from build123d import *

# Parameters (mm, degrees)
F0_W         = 70.9387809038
F0_H         = 53.9411939681
F1_DEPTH     = 38.1
F2_T         = -2.54
F3_R         = 5.08
F4_T1_DEPTH  = 43.7811939681
F4_T3_DEPTH  = 45.72
F4_S7_W      = 5.08
F4_S7_H      = 5.08
F4_T8_DEPTH  = 5.08
F4_S13_W     = 5.08
F4_S13_H     = 5.08
F4_T14_DEPTH = 5.08
F4_T18_ANGLE = 90
F4_T20_ANGLE = 90


# Not quite as in the source:
# - a fillet or chamfer that OpenCascade refuses, or shapes differently, is made with other operations: its cross-section is extruded or revolved along the edge and cut away or added


with BuildPart() as f1:
    # F0 (on Top) → F1 (new body)
    with BuildSketch(Plane.XY):
        Rectangle(F0_W, F0_H)
    extrude(amount=F1_DEPTH)

    # F2
    f2_openings = [f1.faces().sort_by_distance(p)[0] for p in [
        (0, 0, 38.1),
    ]]
    offset(amount=F2_T, openings=f2_openings)

    # F3
    f3_edges = [f1.edges().sort_by_distance(p)[0] for p in [
        (0, 26.970597, 0),
        (0, -26.970597, 0),
        (-35.46939, 26.970597, 19.05),
        (35.46939, -26.970597, 19.05),
    ]]
    fillet(f3_edges, radius=F3_R)

    # F4: fillet of radius 5.08 on 3 edges, made by hand

    # F4_s2 → F4_t1 (cut)
    with BuildSketch(Plane.XZ.offset(-21.890596984)):
        with BuildLine():
            ThreePointArc((30.3893904519, 0), (33.9814929003, 1.4878975516), (35.4693904519, 5.08))
            Line((35.4693904519, 5.08), (35.4693904519, 0))
            Line((35.4693904519, 0), (30.3893904519, 0))
        make_face()
        with BuildLine():
            ThreePointArc((-35.4693904519, 5.08), (-33.9814929003, 1.4878975516), (-30.3893904519, 0))
            Line((-30.3893904519, 0), (-35.4693904519, 0))
            Line((-35.4693904519, 0), (-35.4693904519, 5.08))
        make_face()
    extrude(amount=F4_T1_DEPTH, mode=Mode.SUBTRACT)

    # F4_s4 → F4_t3 (cut)
    with BuildSketch(Plane.XY.offset(5.08)):
        with BuildLine():
            ThreePointArc((-30.3893904519, -26.970596984), (-33.9814929003, -25.4826994325), (-35.4693904519, -21.890596984))
            Line((-35.4693904519, -21.890596984), (-35.4693904519, -26.970596984))
            Line((-35.4693904519, -26.970596984), (-30.3893904519, -26.970596984))
        make_face()
        with BuildLine():
            ThreePointArc((35.4693904519, 21.890596984), (33.9814929003, 25.4826994325), (30.3893904519, 26.970596984))
            Line((30.3893904519, 26.970596984), (35.4693904519, 26.970596984))
            Line((35.4693904519, 26.970596984), (35.4693904519, 21.890596984))
        make_face()
    extrude(amount=F4_T3_DEPTH, mode=Mode.SUBTRACT)


with BuildPart() as f4_tool6:
    # F4_s7 → F4_t8 (new body)
    with BuildSketch(Plane.YZ.offset(-30.3893904519)):
        with Locations((24.430596984, 2.54)):
            Rectangle(F4_S7_W, F4_S7_H)
    extrude(amount=-F4_T8_DEPTH)

    # F4_s9 → F4_t10 (revolve, cut)
    with BuildSketch(Plane(origin=(-30.3893904519, 21.890596984, 5.08), x_dir=(0, -0.7071067812, 0.7071067812), z_dir=(0, -0.7071067812, -0.7071067812))):
        with BuildLine():
            ThreePointArc((0, -5.08), (5.08, 0), (0, 5.08))
            Line((0, 5.08), (0, -5.08))
        make_face()
    revolve(axis=Axis((-30.3893904519, 21.890596984, 5.08), (-1, 0, 0)), mode=Mode.SUBTRACT)


with BuildPart() as f1_1:
    add(f1.part)

    # F4_t5: cut F4_tool6
    add(f4_tool6.part, mode=Mode.SUBTRACT)


with BuildPart() as f4_tool12:
    # F4_s13 → F4_t14 (new body)
    with BuildSketch(Plane.XY.offset(5.08)):
        with Locations((32.9293904519, -24.430596984)):
            Rectangle(F4_S13_W, F4_S13_H)
    extrude(amount=-F4_T14_DEPTH)

    # F4_s15 → F4_t16 (revolve, cut)
    with BuildSketch(Plane(origin=(30.3893904519, -21.890596984, 5.08), x_dir=(-0.7071067812, 0.7071067812, 0), z_dir=(-0.7071067812, -0.7071067812, 0))):
        with BuildLine():
            ThreePointArc((0, -5.08), (5.08, 0), (0, 5.08))
            Line((0, 5.08), (0, -5.08))
        make_face()
    revolve(axis=Axis((30.3893904519, -21.890596984, 5.08), (0, 0, -1)), mode=Mode.SUBTRACT)


with BuildPart() as f1_2:
    add(f1_1.part)

    # F4_t11: cut F4_tool12
    add(f4_tool12.part, mode=Mode.SUBTRACT)

    # F4_s17 → F4_t18 (revolve, cut)
    with BuildSketch(Plane.XY.offset(5.08)):
        with BuildLine():
            ThreePointArc((-35.4693904519, -21.890596984), (-33.9814929003, -25.4826994325), (-30.3893904519, -26.970596984))
            Line((-30.3893904519, -26.970596984), (-35.4693904519, -26.970596984))
            Line((-35.4693904519, -26.970596984), (-35.4693904519, -21.890596984))
        make_face()
    revolve(axis=Axis((-35.4693904519, -21.890596984, 5.08), (1, 0, 0)), revolution_arc=F4_T18_ANGLE, mode=Mode.SUBTRACT)

    # F4_s19 → F4_t20 (revolve, cut)
    with BuildSketch(Plane.XY.offset(5.08)):
        with BuildLine():
            ThreePointArc((35.4693904519, 21.890596984), (33.9814929003, 25.4826994325), (30.3893904519, 26.970596984))
            Line((30.3893904519, 26.970596984), (35.4693904519, 26.970596984))
            Line((35.4693904519, 26.970596984), (35.4693904519, 21.890596984))
        make_face()
    revolve(axis=Axis((35.4693904519, 21.890596984, 5.08), (-1, 0, 0)), revolution_arc=F4_T20_ANGLE, mode=Mode.SUBTRACT)


solid = f1_2.part
Geometry check sheet. Reference: the model listing, model coordinates, mm. A direction names the side the tool comes from. Coordinates: 2 decimals unless noted, no trailing zeros. Order: outer loops, then holes, each group sorted by start corner. A loop starts at its lowest first (then second) coordinate and runs counter-clockwise, first axis right, second up. Notation, with made-up numbers: (-33, 73) -> (15, 73) arc R20 ccw to (15, 110) -> close; hole circle Ø9 at (68.5, 15). An arc over 180 degrees is marked (long way). Use a Markdown table: item, result. Add a question column.
1. Mould release check, pull along X, two halves, no side actions. Record for faces 3 (the face through (-34.021, 0.306, 1.528)), 4 (the face through (34.021, 25.443, 21.359)), 5 (the face through (32.929, 0, 20)): pulls with the +X half, pulls with the -X half, needs draft (parallel to the pull), parting line crosses it, or undercut.
2. Set-up check for faces 1 (the face through (-34.021, 25.443, 21.821)), 2 (the face through (0, 0, 2.54)): record each of +Z, -Z, +X, -X, +Y, -Y from which the full face is reachable in a straight line by a thin tool's end or side.
3. Go/stop test with a flat-tipped pin: pin 1 Ø1.5 at (x, y) = (-3.5, -6) entering from +Z. Record where the tip stops, or that it passes through.
4. Cross-section at C-C (y = -11.5). Enter the section's corners in (x, z), and give its area (3 significant figures).
5. Cross-section at B-B (x = -23). Enter the section's corners in (y, z).
6. Cross-section at A-A (z = 25.5). Enter the section's corners in (x, y), and give its area (3 significant figures).
7. Material ranges on L1, parallel to Y at x = 1, z = 16; L2, parallel to X at y = -15.5, z = 35; L3, parallel to Z at x = -29, y = 9, recorded low to high.
Filled sheet:
| question | item | result |
|---|---|---|
| 1 | face 3 | pulls with the -X half |
| 1 | face 4 | pulls with the +X half |
| 1 | face 5 | undercut |
| 2 | face 1 | +Z, -Z, -X, +Y |
| 2 | face 2 | +Z |
| 3 | pin 1 | z = 2.54 |
| 4 | outline | (-35.47, 5.08) arc R5.08 ccw to (-30.39, 0) -> (30.39, 0) arc R5.08 ccw to (35.47, 5.08) -> (35.47, 38.1) -> (32.93, 38.1) -> (32.93, 2.54) -> (-32.93, 2.54) -> (-32.93, 38.1) -> (-35.47, 38.1) -> close |
| 4 | area | 350 mm2 |
| 5 | outline | (-26.97, 5.08) arc R5.08 ccw to (-21.89, 0) -> (21.89, 0) arc R5.08 ccw to (26.97, 5.08) -> (26.97, 38.1) -> (24.43, 38.1) -> (24.43, 2.54) -> (-24.43, 2.54) -> (-24.43, 38.1) -> (-26.97, 38.1) -> close |
| 6 | outline | (-35.47, -21.89) arc R5.08 ccw to (-30.39, -26.97) -> (30.39, -26.97) arc R5.08 ccw to (35.47, -21.89) -> (35.47, 21.89) arc R5.08 ccw to (30.39, 26.97) -> (-30.39, 26.97) arc R5.08 ccw to (-35.47, 21.89) -> close; hole (-32.93, -24.43) -> (32.93, -24.43) -> (32.93, 24.43) -> (-32.93, 24.43) -> close |
| 6 | area | 586 mm2 |
| 7 | L1 | -26.97 to -24.43, 24.43 to 26.97 |
| 7 | L2 | -35.47 to -32.93, 32.93 to 35.47 |
| 7 | L3 | 0 to 2.54 |
